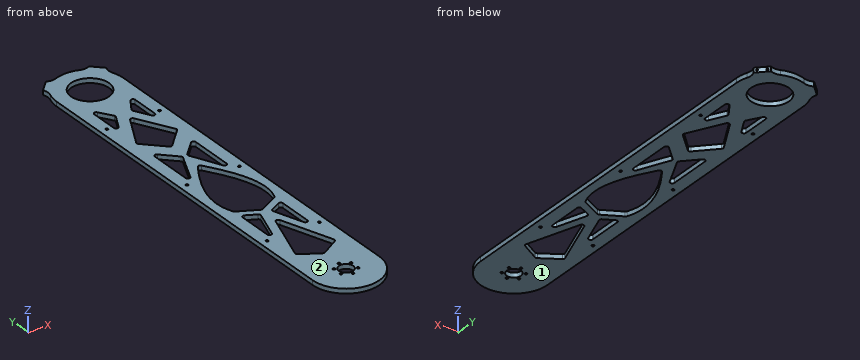
```python
from build123d import *

# Parameters (mm, degrees)
SKETCH2_R                            = 10
SKETCH2_R_2                          = 1.65
BOSS_EXTRUDE1_DEPTH                  = 6.35
CUT_EXTRUDE1_DEPTH                   = 10
FILLET3_R                            = 3
SKETCH5_R                            = 1.75
CUT_EXTRUDE2_DEPTH                   = 549.511460792
SKETCH6_R                            = 26.5
CUT_EXTRUDE3_DEPTH                   = 10
BOSS_EXTRUDE2_START                  = -6.35
BOSS_EXTRUDE2_DEPTH                  = 6.35
TAP_DRILL_FOR_M3X0_5_TAP1_AT_2_COUNT = 2
TAP_DRILL_FOR_M3X0_5_TAP1_AT_2_PITCH = 12
CIRPATTERN2_COUNT                    = 2
CIRPATTERN2_ANGLE                    = 90


with BuildPart() as part:
    # Sketch2 → Boss-Extrude1 (new body)
    with BuildSketch(Plane.XY):
        with BuildLine():
            Line((-46.5, 0), (-46.5, 500))
            ThreePointArc((-46.5, 500), (0, 546.5), (46.5, 500))
            Line((46.5, 500), (46.5, 0))
            ThreePointArc((46.5, 0), (0, -46.5), (-46.5, 0))
        make_face()
        Circle(SKETCH2_R, mode=Mode.SUBTRACT)
        with Locations((0, 13.75)):
            Circle(SKETCH2_R_2, mode=Mode.SUBTRACT)
        with Locations((11.907849302, 6.875)):
            Circle(SKETCH2_R_2, mode=Mode.SUBTRACT)
        with Locations((11.907849302, -6.875)):
            Circle(SKETCH2_R_2, mode=Mode.SUBTRACT)
        with Locations((0, -13.75)):
            Circle(SKETCH2_R_2, mode=Mode.SUBTRACT)
        with Locations((-11.907849302, -6.875)):
            Circle(SKETCH2_R_2, mode=Mode.SUBTRACT)
        with Locations((-11.907849302, 6.875)):
            Circle(SKETCH2_R_2, mode=Mode.SUBTRACT)
    extrude(amount=BOSS_EXTRUDE1_DEPTH)

    # Sketch4 → Cut-Extrude1 (cut)
    with BuildSketch(Plane.XY.offset(6.35)):
        Polygon((28.005258112, 59.37595418), (0, 42.411661153), (-28.005258112, 59.37595418), (0, 141.693437584), align=None)
        Polygon((-7.5, 156.905935087), (-28.005258112, 96.633637735), (-28.005258112, 167.582877854), align=None)
        Polygon((28.005258112, 167.582877854), (7.5, 156.905935087), (28.005258112, 96.633637735), align=None)
        with BuildLine():
            Line((0, 164.275138905), (28.550546746, 179.141206521))
            add(Edge.make_bspline(
                [(28.550546746, 179.141206521), (45.32025339, 216.985654627), (19.430092874, 259.790255689), (0, 290.025756679)],
                knots=[0, 0, 0, 0, 1, 1, 1, 1], degree=3))
            add(Edge.make_bspline(
                [(-28.550546746, 179.141206521), (-45.32025339, 216.985654627), (-19.430092874, 259.790255689), (0, 290.025756679)],
                knots=[0, 0, 0, 0, 1, 1, 1, 1], degree=3))
            Line((-28.550546746, 179.141206521), (0, 164.275138905))
        make_face()
        Polygon((28.550546746, 259.58677623), (3, 314.938284003), (28.550546746, 340.793051053), align=None)
        Polygon((-3, 314.938284003), (-28.550546746, 340.793051053), (-28.550546746, 259.58677623), align=None)
        Polygon((0, 423.142843498), (-28.550546746, 369.246205395), (0, 340.355718526), (28.550546746, 369.246205395), align=None)
        Polygon((-28.550546746, 462.095190817), (-28.550546746, 401.290241252), (-11, 434.421497018), align=None)
        Polygon((28.550546746, 401.290241252), (11, 434.421497018), (28.550546746, 462.095190817), align=None)
    extrude(amount=-CUT_EXTRUDE1_DEPTH, mode=Mode.SUBTRACT)

    # Fillet3
    fillet3_edges = [part.edges().sort_by_distance(p)[0] for p in [
        (-11, 434.421497018, 3.175),
        (-28.550546746, 401.290241252, 3.175),
        (28.550546746, 401.290241252, 3.175),
        (11, 434.421497018, 3.175),
        (28.550546746, 462.095190817, 3.175),
        (-28.550546746, 462.095190817, 3.175),
        (0, 423.142843498, 3.175),
        (-28.550546746, 369.246205395, 3.175),
        (28.550546746, 369.246205395, 3.175),
        (0, 340.355718526, 3.175),
        (28.550546746, 340.793051053, 3.175),
        (-28.550546746, 340.793051053, 3.175),
        (-3, 314.938284003, 3.175),
        (3, 314.938284003, 3.175),
        (28.550546746, 259.58677623, 3.175),
        (-28.550546746, 259.58677623, 3.175),
        (28.550546746, 179.141206521, 3.175),
        (0, 290.025756679, 3.175),
        (-28.550546746, 179.141206521, 3.175),
        (0, 164.275138905, 3.175),
        (-28.005258112, 96.633637735, 3.175),
        (28.005258112, 96.633637735, 3.175),
        (7.5, 156.905935087, 3.175),
        (-28.005258112, 167.582877854, 3.175),
        (28.005258112, 167.582877854, 3.175),
        (0, 141.693437584, 3.175),
        (28.005258112, 59.37595418, 3.175),
        (-28.005258112, 59.37595418, 3.175),
        (0, 42.411661153, 3.175),
        (-7.5, 156.905935087, 3.175),
    ]]
    fillet(fillet3_edges, radius=FILLET3_R)

    # Sketch5 → Cut-Extrude2 (cut, through all)
    with BuildSketch(Plane.XY.offset(6.35)):
        with Locations((36.5, 103.175)):
            Circle(SKETCH5_R)
        with Locations(Location((-36.5, 103.175, 0), (0, 0, 180))):
            Circle(SKETCH5_R)
        with Locations(Location((36.5, 259.525, 0), (0, 0, 180))):
            Circle(SKETCH5_R)
        with Locations((-36.5, 259.525)):
            Circle(SKETCH5_R)
        with Locations((36.5, 415.875)):
            Circle(SKETCH5_R)
        with Locations(Location((-36.5, 415.875, 0), (0, 0, 180))):
            Circle(SKETCH5_R)
    extrude(amount=-CUT_EXTRUDE2_DEPTH, mode=Mode.SUBTRACT)

    # Sketch6 → Cut-Extrude3 (cut)
    with BuildSketch(Plane.XY.offset(6.35)):
        with Locations((0, 500)):
            Circle(SKETCH6_R)
    extrude(amount=-CUT_EXTRUDE3_DEPTH, mode=Mode.SUBTRACT)

    # Sketch7 → Boss-Extrude2 (add)
    with BuildSketch(Plane.XY.offset(6.35).offset(BOSS_EXTRUDE2_START)):
        with BuildLine():
            Line((44.110383395, 529.968247771), (29.968247771, 544.110383395))
            ThreePointArc((29.968247771, 544.110383395), (23.286397782, 542.399293624), (16.474718596, 543.483717035))
            ThreePointArc((16.474718596, 543.483717035), (32.880465325, 532.880465325), (43.483717035, 516.474718596))
            ThreePointArc((43.483717035, 516.474718596), (42.399293624, 523.286397782), (44.110383395, 529.968247771))
        make_face()
    boss_extrude2 = extrude(amount=BOSS_EXTRUDE2_DEPTH)

    # Sketch9 → Tap Drill for M3x0.5 Tap1 (revolve, cut)
    with BuildSketch(Plane(origin=(32.796674896, 541.28195627, 3.175), x_dir=(-0.7071067811865481, 0.7071067811865469, 0), z_dir=(0, 0, 1))):
        Polygon((0, 0), (0, 5.751075774), (1.25, 5), (1.25, 0), align=None)
    tap_drill_for_m3x0_5_tap1 = revolve(axis=Axis((37.286802956, 545.772084331, 3.175), (-0.7071067811865468, -0.7071067811865482, 0)), mode=Mode.SUBTRACT)

    # Tap Drill for M3x0.5 Tap1 at 2: Tap Drill for M3x0.5 Tap1 ×2
    with Locations(*[Vector(0.7071067811865482, -0.7071067811865468, 0) * (i * TAP_DRILL_FOR_M3X0_5_TAP1_AT_2_PITCH) for i in range(1, TAP_DRILL_FOR_M3X0_5_TAP1_AT_2_COUNT)]):
        add(tap_drill_for_m3x0_5_tap1, mode=Mode.SUBTRACT)

    # CirPattern2: Boss-Extrude2, Tap Drill for M3x0.5 Tap1 ×2 about axis
    cirpattern2_axis = Axis((0, 500, 0), (0, 0, 1))
    add([boss_extrude2.rotate(cirpattern2_axis, i * CIRPATTERN2_ANGLE / (CIRPATTERN2_COUNT - 1)) for i in range(1, CIRPATTERN2_COUNT)])
    add([tap_drill_for_m3x0_5_tap1.rotate(cirpattern2_axis, i * CIRPATTERN2_ANGLE / (CIRPATTERN2_COUNT - 1)) for i in range(1, CIRPATTERN2_COUNT)], mode=Mode.SUBTRACT)

    # CirPattern2 copy 1 sketch → CirPattern2 copy 1 (revolve, cut)
    with BuildSketch(Plane(origin=(-32.796674896, 541.28195627, 3.175), x_dir=(-0.7071067811865445, -0.7071067811865506, 0), z_dir=(0, 0, 1))):
        Polygon((0, 0), (0, 5.751075774), (1.25, 5), (1.25, 0), align=None)
    revolve(axis=Axis((-37.286802956, 545.772084331, 3.175), (0.7071067811865507, -0.7071067811865444, 0)), mode=Mode.SUBTRACT)


solid = part.part
```
The model under review builds one solid part; all positions refer to its coordinate system, in mm. Face numbers are marked on the shaded views. Give positions to 0.01 mm unless a question says otherwise; leave off trailing zeros.
(1) For P1, Ø4, axis at x = -26.5, y = 318, coming from the -Z side, flat-tipped, find the tip position at first contact; note if it passes through.
(2) To check wall thickness, follow L1, parallel to X at y = 58.5, z = 4.25; L2, parallel to X at y = 414, z = 0.5; L3, parallel to X at y = 62, z = 3.25. State the ranges of each line that lie inside material, in increasing order.
(3) The part is to be moulded in two halves that separate along Z. For the marked faces 1 and 2, say which applies: released by +Z, released by -Z, zero draft, split by the parting line, or undercut.
Returned:
1. P1: passes through
2. L1: x = -46.5 to -26.44, 26.44 to 46.5
2. L2: x = -46.5 to -28.55, -21.82 to -4.84, 4.84 to 21.82, 28.55 to 46.5
2. L3: x = -46.5 to -27.11, 27.11 to 46.5
3. face 1: released by -Z
3. face 2: released by +Z
